The figure shows three views and two pictorial views of one solid part (mm, origin at its lowest corner). Answer the questions. A direction names the side the tool comes from. Coordinates: 2 decimals unless noted, no trailing zeros. Write each loop counter-clockwise with the first axis right and the second up, starting at its lowest first coordinate (ties: lowest second). Pieces come first, ordered by that corner, then holes.
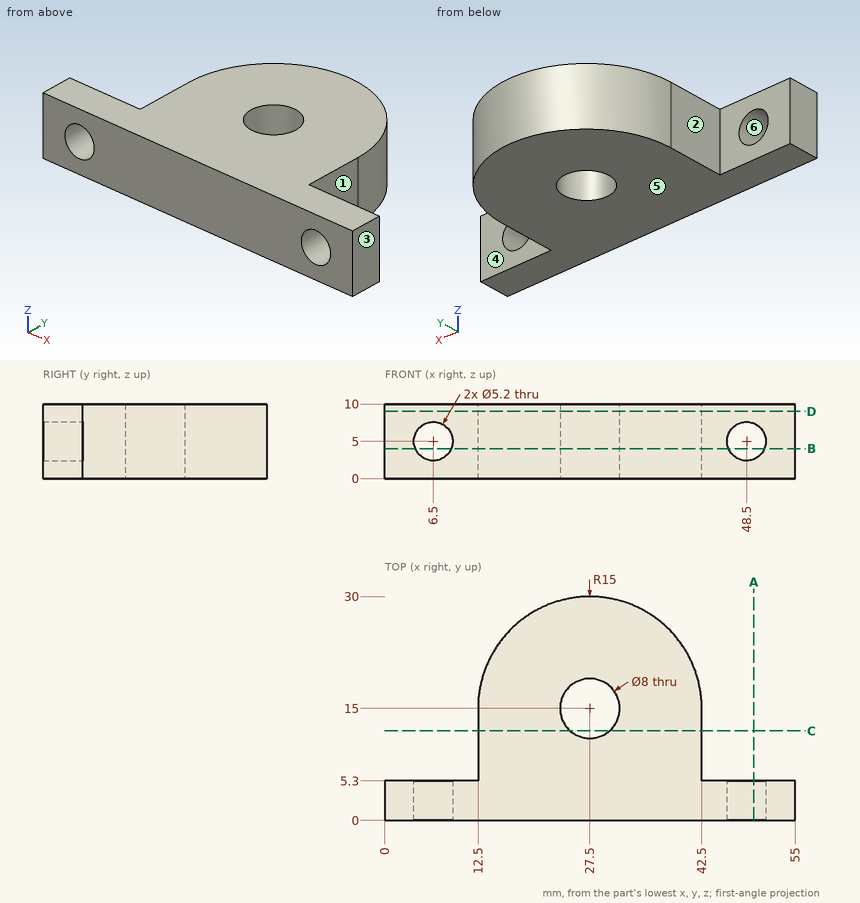
1. A tool of negligible diameter and unlimited length cuts with its end or side. For the marked faces 1, 2 and 3, from which of +Z, -Z, +X, -X, +Y, -Y can it reach the whole face along a straight path? Write none if from no direction.
Results found:
face 1: +Z, -Z, +X, +Y
face 2: +Z, -Z, -X, +Y
face 3: +Z, -Z, +X, +Y, -Y
2. Section C-C on y = 12 is taken. Give the vertices of the cut face in (x, z).
Results found:
outline: (12.5, 0) - (24.85, 0) - (24.85, 10) - (12.5, 10) - close; (30.15, 0) - (42.5, 0) - (42.5, 10) - (30.15, 10) - close
3. Section A-A on x = 49.5 is taken. Give the vertices of the cut face in (y, z).
Results found:
outline: (0, 0) - (5.3, 0) - (5.3, 2.6) - (0, 2.6) - close; (0, 7.4) - (5.3, 7.4) - (5.3, 10) - (0, 10) - close
4. Section D-D on z = 9 is taken. Give the vertices of the cut face in (x, y).
Results found:
outline: (0, 0) - (55, 0) - (55, 5.3) - (42.5, 5.3) - (42.5, 15) arc R15 ccw to (12.5, 15) - (12.5, 5.3) - (0, 5.3) - close; hole circle Ø8 at (27.5, 15)
5. Section B-B on z = 4 is taken. Give the vertices of the cut face in (x, y), then the cut area to 3 significant figures.
Results found:
outline: (0, 0) - (4.1, 0) - (4.1, 5.3) - (0, 5.3) - close; (8.9, 0) - (46.1, 0) - (46.1, 5.3) - (42.5, 5.3) - (42.5, 15) arc R15 ccw to (12.5, 15) - (12.5, 5.3) - (8.9, 5.3) - close; (50.9, 0) - (55, 0) - (55, 5.3) - (50.9, 5.3) - close; hole circle Ø8 at (27.5, 15)
area: 835 mm2
6. For a pull along Z with two mould halves and no side action, classify the marked faces 4, 5 and 6 as pulls with the +Z half, pulls with the -Z half, needs draft (parallel to the pull), parting line crosses it, or undercut.
Results found:
face 4: needs draft
face 5: pulls with the -Z half
face 6: undercut
7. Find the intervals of material crossed by L1, parallel to X at y = 2.45, z = 5; L2, parallel to Y at x = 27.5, z = 7.5; L3, parallel to Z at x = 48.5, y = 1.5, in increasing order.
Results found:
L1: x = 0 to 3.9, 9.1 to 45.9, 51.1 to 55
L2: y = 0 to 11, 19 to 30
L3: z = 0 to 2.4, 7.6 to 10
8. Flat-ended cylindrical pins translate along their axes: P1, Ø4, axis at x = 14.5, z = 6, coming from the +Y side; P2, Ø1, axis at x = 44.5, z = 7.5, coming from the +Y side; P3, Ø4, axis at y = 8, z = 3, coming from the -X side. Find the tip coordinate at first contact, or state that the pin passes through.
Results found:
P1: stops at y = 25.2
P2: stops at y = 5.3
P3: stops at x = 12.5
